Work out the finished part from the listing and answer in its coordinate system (mm). Face numbers are marked on the shaded views. A direction names the side the tool comes from. Give positions to 0.01 mm unless a question says otherwise; leave off trailing zeros. Order: outer loops, then holes, each group sorted by start corner. A loop starts at its lowest first (then second) coordinate and runs counter-clockwise, first axis right, second up. Notation, with made-up numbers: (75, -34) -> (107, -34) arc R10 cw to (107, -28) -> close; hole circle Ø1 at (-2.5, -19). An arc over 180 degrees is marked (long way). Answer as CSV lines item,"result". Start each with the question number.
1. A cutting plane is placed at A-A (z = 44.5). Give the vertices of the cut face in (x, y), then the cut area to 3 significant figures.
2. Find the intervals of material crossed by L1, parallel to X at y = -39.5, z = 51; L2, parallel to Y at x = -21.5, z = 53; L3, parallel to Z at x = 4.5, y = -29, in increasing order.
3. Flat-ended cylindrical pins translate along their axes: pin 1 (2 mm diameter, centred on x = 29.5, z = 38.5, fed in from +Y); pin 2 (2 mm diameter, centred on x = 30, z = 37.5, fed in from -Y); pin 3 (2.5 mm diameter, centred on y = -45, z = 22.5, fed in from -X). Find the tip coordinate at first contact, or state that the pin passes through.
4. For a pull along X with two mould halves and no side action, classify the marked faces 3, 4 and 5 as released by +X, released by -X, zero draft, split by the parting line, or undercut.
5. A cutting plane is placed at B-B (y = 19.5). Give the vertices of the cut face in (x, z).
6. A cutting plane is placed at D-D (z = 60). Give the vertices of the cut face in (x, y).
7. A cutting plane is placed at C-C (x = -11.5). Give the vertices of the cut face in (y, z), then the cut area to 3 significant figures.
8. For the marked faces 1 and 2, determine the directions among +Z, -Z, +X, -X, +Y, -Y from which every point of the face is accessible in a straight line to the end or side of a thin tool.
from build123d import *

# Parameters (mm, degrees)
BOX038_W     = 10
BOX038_H     = 58
BOX038_DEPTH = 25
FILLET007_R  = 4
BOX035_W     = 10
BOX035_H     = 58
BOX035_DEPTH = 25
BOX034_W     = 56
BOX034_H     = 85
BOX034_DEPTH = 40
THICKNESS_T  = 2.5
SKETCH_W     = 6
SKETCH_H     = 3
PAD006_DEPTH = 5


with BuildPart() as fillet007:
    # Box038 → Box038 (new body)
    with BuildSketch(Plane(origin=(23, -30, 25), x_dir=(1, 0, 0), z_dir=(0, 0, 1))):
        with Locations((5, 29)):
            Rectangle(BOX038_W, BOX038_H)
    extrude(amount=BOX038_DEPTH)

    # Fillet007
    fillet007_edges = [fillet007.edges().sort_by_distance(p)[0] for p in [
        (28, -30, 50),
        (28, 28, 50),
    ]]
    fillet(fillet007_edges, radius=FILLET007_R)


with BuildPart() as cubo029:
    # Box035 → Box035 (new body)
    with BuildSketch(Plane(origin=(-36, -30, 25), x_dir=(1, 0, 0), z_dir=(0, 0, 1))):
        with Locations((5, 29)):
            Rectangle(BOX035_W, BOX035_H)
    extrude(amount=BOX035_DEPTH)


with BuildPart() as obj1:
    # Box034 → Box034 (new body)
    with BuildSketch(Plane(origin=(-31, -46, 38), x_dir=(1, 0, 0), z_dir=(0, 0, 1))):
        with Locations((28, 42.5)):
            Rectangle(BOX034_W, BOX034_H)
    extrude(amount=BOX034_DEPTH)

    # Thickness
    thickness_openings = [obj1.faces().sort_by_distance(p)[0] for p in [
        (-3, -3.5, 38),
    ]]
    offset(amount=THICKNESS_T, openings=thickness_openings)


with BuildPart() as obj1_1:
    # Thickness placement: moved
    add(obj1.part.moved(Location((2, 2, -13))))

    # Cut045: cut Cubo029
    add(cubo029.part, mode=Mode.SUBTRACT)


with BuildPart() as obj1_2:
    # Cut045 placement: moved
    add(obj1_1.part.moved(Location((1, 1, 0))))

    # Sketch → Pad006 (new body)
    with BuildSketch(Plane(origin=(1, 1, 25), x_dir=(1, 0, 0), z_dir=(0, 0, -1))):
        with Locations((0, 45.5)):
            Rectangle(SKETCH_W, SKETCH_H)
        with Locations((0, -42.5)):
            Rectangle(SKETCH_W, SKETCH_H)
    extrude(amount=PAD006_DEPTH)

    # Cut048: cut Fillet007
    add(fillet007.part, mode=Mode.SUBTRACT)


solid = obj1_2.part
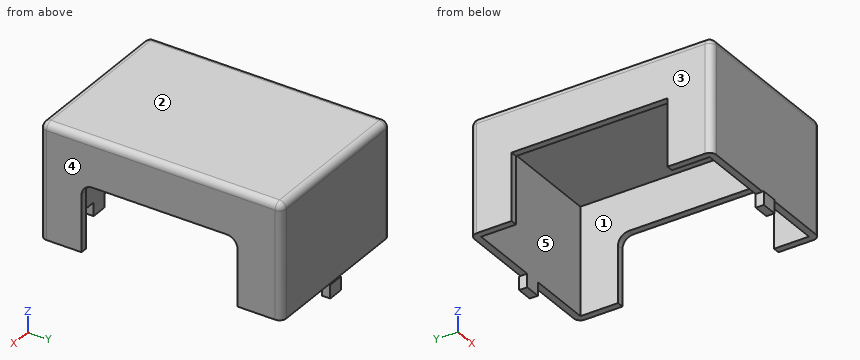
Answer sheet:
1,outline,"(-30.5, -43) arc R2.5 ccw to (-28, -45.5) -> (28, -45.5) arc R2.5 ccw to (30.5, -43) -> (30.5, -30) -> (28, -30) -> (28, -43) -> (-28, -43) -> (-28, -29) -> (-30.5, -29) -> close; (-30.5, 29) -> (-28, 29) -> (-28, 42) -> (28, 42) -> (28, 28) -> (30.5, 28) -> (30.5, 42) arc R2.5 ccw to (28, 44.5) -> (-28, 44.5) arc R2.5 ccw to (-30.5, 42) -> close"
1,area,"435 mm^2"
2,L1,"x = -30.5 to -28, 28 to 30.5"
2,L2,"y = -45.5 to -43, 42 to 44.5"
2,L3,"z = 65 to 67.5"
3,pin 1,"stops at y = 44.45"
3,pin 2,"stops at y = -45.29"
3,pin 3,"stops at x = -2"
4,face 3,"released by -X"
4,face 4,"released by +X"
4,face 5,"undercut"
5,outline,"(-30.5, 50) -> (-28, 50) -> (-28, 65) -> (28, 65) -> (28, 50) -> (30.5, 50) -> (30.5, 65) arc R2.5 ccw to (28, 67.5) -> (-28, 67.5) arc R2.5 ccw to (-30.5, 65) -> close"
6,outline,"(-30.5, -43) arc R2.5 ccw to (-28, -45.5) -> (28, -45.5) arc R2.5 ccw to (30.5, -43) -> (30.5, 42) arc R2.5 ccw to (28, 44.5) -> (-28, 44.5) arc R2.5 ccw to (-30.5, 42) -> close; hole (-28, -43) -> (28, -43) -> (28, 42) -> (-28, 42) -> close"
7,outline,"(-45.5, 25) -> (-43, 25) -> (-43, 65) -> (42, 65) -> (42, 25) -> (44.5, 25) -> (44.5, 65) arc R2.5 ccw to (42, 67.5) -> (-43, 67.5) arc R2.5 ccw to (-45.5, 65) -> close"
7,area,"422 mm^2"
8,face 1,"-Z"
8,face 2,"+Z, +X, -X, +Y, -Y"
